Build history of the part. All positions in model axes, mm. A direction names the side the tool comes from. Give positions to 0.01 mm unless a question says otherwise; leave off trailing zeros. Loops run counter-clockwise (first coordinate to the right, second up) from the corner with the lowest first, then second, coordinate; pieces in that order, holes last. Notation, with made-up numbers: M 49.25,-35.5 L 101.25,-35.5 A17 cw 101.25,-9.5 Z; hole C 69.5,-15.5 d1. An arc over 180 degrees is marked long. Answer in a Markdown table with one row per item. Add a question column.
```python
from build123d import *

# Parameters (mm, degrees)
F1_DEPTH = 533.4
F4_W     = 10.16
F4_H     = 38.1
F5_DEPTH = 38.1
F6_R     = 5.07999
F3_W     = 20.32
F3_H     = 279.4
F7_DEPTH = 12.7
F8_R     = 5.08


# Not quite as in the source:
# - a fillet or chamfer is up to 0.001 mm smaller than in the source, because OpenCascade refuses the exact size


with BuildPart() as f1:
    # F0 (on Top) → F1 (new body)
    with BuildSketch(Plane.XY):
        with BuildLine():
            Line((63.5, 25.4), (-76.2, 25.4))
            Line((-76.2, 25.4), (-76.2, 12.7))
            ThreePointArc((-76.2, 12.7), (-72.4802561211, 3.7197438789), (-63.5, 0))
            Line((-63.5, 0), (63.5, 0))
            ThreePointArc((63.5, 0), (72.4802561211, 3.7197438789), (76.2, 12.7))
            ThreePointArc((76.2, 12.7), (72.4802561211, 21.6802561211), (63.5, 25.4))
        make_face()
    extrude(amount=F1_DEPTH)

    # F4 (on face) → F5 (join, through all)
    with BuildSketch(Plane.XZ):
        with Locations((40.64, 336.55)):
            Rectangle(F4_W, F4_H)
        with Locations((40.64, 171.45)):
            Rectangle(F4_W, F4_H)
    extrude(amount=F5_DEPTH)

    # F6 (radius 5.08 in the source; OpenCascade refuses exactly that, so slightly less here)
    f6_edges = [f1.edges().sort_by_distance(p)[0] for p in [
        (35.56, -19.05, 355.6),
        (45.72, -19.05, 355.6),
        (45.72, -19.05, 317.5),
        (35.56, -19.05, 317.5),
        (35.56, -19.05, 190.5),
        (45.72, -19.05, 190.5),
        (35.56, -19.05, 152.4),
        (45.72, -19.05, 152.4),
    ]]
    fillet(f6_edges, radius=F6_R)

    # F3 (on offset) → F7 (join)
    with BuildSketch(Plane.XZ.offset(38.1)):
        with Locations((40.64, 266.7)):
            Rectangle(F3_W, F3_H)
    extrude(amount=F7_DEPTH)

    # F8
    f8_edges = [f1.edges().sort_by_distance(p)[0] for p in [
        (40.64, -50.8, 406.4),
        (30.48, -50.8, 266.7),
        (50.8, -50.8, 266.7),
        (40.64, -50.8, 127),
    ]]
    fillet(f8_edges, radius=F8_R)


solid = f1.part
```
(1) Slice it at D-D, the plane x = 18. Give the cut face in (y, z).
(2) Pin check, flat tips, straight feed: pin 1 (4 mm diameter, centred on y = -42.5, z = 285, fed in from -X); pin 2 (6 mm diameter, centred on y = -41, z = 221, fed in from +X); pin 3 (4 mm diameter, centred on x = 39.5, y = -40.5, fed in from -Z). Stop position of each tip, or through.
(3) Tool access for faces 5 (the flat face through (45.72, -19, 336)), 6 (the flat face through (35.56, -19, 171)), 7 (the flat face through (41, -50.8, 269)): list every direction of +Z, -Z, +X, -X, +Y, -Y with a clear straight run to the whole face (end or side of a thin tool).
(4) Slice it at C-C, the plane z = 345. Give the cut face in (x, y), then the cut area to 3 significant figures.
(5) Wall check: line 1 (Y direction, x = 31, z = 86); line 2 (Z direction, x = 39.5, y = -23); line 3 (X direction, y = -11, z = 323.5). Give the ranges that are in metal, low to high.
(6) Pull direction Z, two halves, no side cores. Call faces 1 (the flat face through (40, -38.1, 269)), 2 (the flat face through (45.72, -19, 171)), 3 (the flat face through (-1, 13, 0)), 4 (the flat face through (-1, 13, 533.4)): +Z half, -Z half, draft (parallel to the pull), parting line (faces both ways), or undercut.
(7) Slice it at B-B, the plane z = 239.5. Give the cut face in (x, y), then the cut area to 3 significant figures.
Solution:
| question | item | result |
|---|---|---|
| 1 | outline | M 0,0 L 25.4,0 L 25.4,533.4 L 0,533.4 Z |
| 2 | pin 1 | x = 30.48 |
| 2 | pin 2 | x = 50.8 |
| 2 | pin 3 | z = 127 |
| 3 | face 5 | +Z, -Z, +X |
| 3 | face 6 | +Z, -Z, -X |
| 3 | face 7 | +Z, -Z, +X, -X, -Y |
| 4 | outline | M -76.2,12.7 A12.7 ccw -63.5,0 L 35.56,0 L 35.56,-38.1 L 30.48,-38.1 L 30.48,-45.72 A5.08 ccw 35.56,-50.8 L 45.72,-50.8 A5.08 ccw 50.8,-45.72 L 50.8,-38.1 L 45.72,-38.1 L 45.72,0 L 63.5,0 A12.7 ccw 63.5,25.4 L -76.2,25.4 Z |
| 4 | area | 4,400 mm^2 |
| 5 | line 1 | 0 to 25.4 |
| 5 | line 2 | 152.53 to 190.37, 317.63 to 355.47 |
| 5 | line 3 | 35.56 to 45.72 |
| 6 | face 1 | undercut |
| 6 | face 2 | draft |
| 6 | face 3 | -Z half |
| 6 | face 4 | +Z half |
| 7 | outline | M -76.2,12.7 A12.7 ccw -63.5,0 L 63.5,0 A12.7 ccw 63.5,25.4 L -76.2,25.4 Z; M 30.48,-45.72 A5.08 ccw 35.56,-50.8 L 45.72,-50.8 A5.08 ccw 50.8,-45.72 L 50.8,-38.1 L 30.48,-38.1 Z |
| 7 | area | 4,010 mm^2 |
